Check sheet for the modelled part. Datum: model origin and axes. Units: mm. A direction names the side the tool comes from. Round coordinates to 2 decimals unless told otherwise and drop trailing zeros. Order: outer loops, then holes, each group sorted by start corner. A loop starts at its lowest first (then second) coordinate and runs counter-clockwise, first axis right, second up. Notation, with made-up numbers: M 28,-25 L 59,-25 A8 cw 59,-16 Z; hole C 8.5,51.5 d8. An arc over 180 degrees is marked long. One line per item, written item: value. Start each with the question number.
(1) Thickness scan on L1, parallel to X at y = 31.75, z = 3.5; L2, parallel to Y at x = 44.45, z = 3; L3, parallel to Z at x = -6, y = 0 (3 decimals). Record the ranges inside material, lowest first.
(2) Release check for a two-part mould opening along Y. For faces 3 (the face through (-44, -32, 6.35)), 4 (the face through (-1, -38.1, 13)), 5 (the face through (44, 32, 6.35)), 6 (the face through (-1, 1, 0)) record: released by +Y, released by -Y, zero draft, split by the parting line, or undercut.
(3) Depth check by flat-ended pin: pin 1 Ø2 at (x, y) = (44.45, 31.75) entering from -Z. Enter the tip coordinate at first touch or a pass-through.
(4) Cross-section at C-C, the plane z = 12.5. Enter the section's corners in (x, y), and give its area (3 significant figures).
(5) Cross-section at D-D, the plane y = 31.75. Enter the section's corners in (x, z), and give its area (3 significant figures).
(6) Access from +Z, -Z, +X, -X, +Y, -Y to the whole of each face (thin tool, end or side, straight path). Record for faces 1 (the face through (-1, 1, 25.4)), 2 (the face through (-45.901, 32.863, 3.131)).
(7) Cross-section at B-B, the plane x = -44.45. Enter the section's corners in (y, z) (3 decimals).
(8) Cross-section at A-A, the plane y = 0. Enter the section's corners in (x, z) (3 decimals).
from build123d import *

# Parameters (mm, degrees)
F0_W     = 101.6
F0_H     = 76.2
F1_DEPTH = 25.4
F2_R     = 6.35
F3_DEPTH = 101.6
F4_R     = 1.8288
F5_DEPTH = 6.35


with BuildPart() as f1:
    # F0 (on Top) → F1 (new body)
    with BuildSketch(Plane.XY):
        Rectangle(F0_W, F0_H)
    extrude(amount=F1_DEPTH)

    # F2 (on face) → F3 (cut)
    with BuildSketch(Plane.YZ.offset(50.8)):
        with Locations((0, 9.525)):
            Circle(F2_R)
    extrude(amount=-F3_DEPTH, mode=Mode.SUBTRACT)

    # F4 (on face) → F5 (cut)
    with BuildSketch(Plane(origin=(0, 0, 0), x_dir=(1, 0, 0), z_dir=(0, 0, -1))):
        with Locations((-44.45, 31.75)):
            Circle(F4_R)
        with Locations((-44.45, -31.75)):
            Circle(F4_R)
        with Locations((44.45, -31.75)):
            Circle(F4_R)
        with Locations((44.45, 31.75)):
            Circle(F4_R)
    extrude(amount=-F5_DEPTH, mode=Mode.SUBTRACT)


solid = f1.part
Values found:
1. L1: -50.8 to -46.28, -42.62 to 42.62, 46.28 to 50.8
1. L2: -38.1 to -33.58, -29.92 to 29.92, 33.58 to 38.1
1. L3: 0 to 3.175, 15.875 to 25.4
2. face 3: undercut
2. face 4: released by -Y
2. face 5: undercut
2. face 6: zero draft
3. pin 1: z = 6.35
4. outline: M -50.8,-38.1 L 50.8,-38.1 L 50.8,-5.61 L -50.8,-5.61 Z; M -50.8,5.61 L 50.8,5.61 L 50.8,38.1 L -50.8,38.1 Z
4. area: 6,600 mm^2
5. outline: M -50.8,0 L -46.28,0 L -46.28,6.35 L -42.62,6.35 L -42.62,0 L 42.62,0 L 42.62,6.35 L 46.28,6.35 L 46.28,0 L 50.8,0 L 50.8,25.4 L -50.8,25.4 Z
5. area: 2,530 mm^2
6. face 1: +Z, +X, -X, +Y, -Y
6. face 2: -Z
7. outline: M -38.1,0 L -33.579,0 L -33.579,6.35 L -29.921,6.35 L -29.921,0 L 29.921,0 L 29.921,6.35 L 33.579,6.35 L 33.579,0 L 38.1,0 L 38.1,25.4 L -38.1,25.4 Z; hole C 0,9.525 d12.7
8. outline: M -50.8,0 L 50.8,0 L 50.8,3.175 L -50.8,3.175 Z; M -50.8,15.875 L 50.8,15.875 L 50.8,25.4 L -50.8,25.4 Z
